Design review of the part built by this model. Coordinates are the model's own, in mm. A direction names the side the tool comes from. Coordinates: 2 decimals unless noted, no trailing zeros. Write each loop counter-clockwise with the first axis right and the second up, starting at its lowest first coordinate (ties: lowest second). Pieces come first, ordered by that corner, then holes.
Q1. Machinability: for faces 4 (the face through (-4, 1, 4)), 5 (the face through (2, 0, -2)), 6 (the face through (1.908, 12.601, -4.458)), 7 (the face through (2, 16, -2)), 8 (the face through (-5, 12, 2)), which of the approach directions +Z, -Z, +X, -X, +Y, -Y give a long, thin tool a straight path to every point of the face, cutting with its end or side? Answer none if there is none.
Q2. Add section B-B, the plane z = 0. Give the boundary of the cut face in (x, y), plus the area to 3 significant figures.
Q3. To check wall thickness, follow probe 1 along Y at (x, z) = (4.5, -5.5); probe 2 along X at (y, z) = (4.25, 0); probe 3 along X at (y, z) = (2.5, 0.5). State the ranges of each line that lie inside material, in increasing order.
Q4. Add section D-D, the plane y = 12. Give the boundary of the cut face in (x, z).
Q5. Add section C-C, the plane x = -5.75. Give the boundary of the cut face in (y, z).
Q6. Add section A-A, the plane x = 0. Give the boundary of the cut face in (y, z), plus the area to 3 significant figures.
Q7. Clearance check with flat-ended pins moving along their axes: pin 1 Ø3 at (x, z) = (0, 0) entering from +Y; pin 2 Ø4 at (y, z) = (7.5, 3) entering from -X; pin 3 Ø3 at (x, y) = (-3.5, 3.5) entering from -Z; pin 4 Ø1.5 at (x, y) = (1.5, 2) entering from -Z. State where each tip first meets the part, or that it passes through.
Q8. The part is to be moulded in two halves that separate along X. For faces 1 (the face through (-4, 8, 4)), 2 (the face through (0.33, 0.493, -7.493)), 3 (the face through (2.11, 8.11, 1.34)), say which applies: +X half, -X half, draft (parallel to the pull), parting line (faces both ways), or undercut.
from build123d import *

# Parameters (mm, degrees)
ESQUISSE1_R                  = 7.5
BOSS_EXTRU_1_DEPTH           = 16
ESQUISSE2_W                  = 2
ESQUISSE2_H                  = 7
ESQUISSE3_R                  = 2.5
ENL_V_MAT_EXTRU_1_DEPTH      = 16
ESQUISSE4_R                  = 2
ENL_V_MAT_EXTRU_2_DEPTH      = 20.19635382
R_P_TITION_CIRCULAIRE1_COUNT = 2
R_P_TITION_CIRCULAIRE1_ANGLE = 90


with BuildPart() as part:
    # Esquisse1 → Boss.-Extru.1 (new body)
    with BuildSketch(Plane(origin=(0, 0, 0), x_dir=(1, 0, 0), z_dir=(0, 1, 0))):
        with Locations(Location((0, 0, 0), (0, 0, 270))):
            Circle(ESQUISSE1_R)
    extrude(amount=BOSS_EXTRU_1_DEPTH)

    # Esquisse2 → Enlèvement de matière-Révolution1 (revolve, cut)
    with BuildSketch(Plane(origin=(0, 0, 0), x_dir=(0, 0, -1), z_dir=(1, 0, 0)), mode=Mode.PRIVATE) as enl_vement_de_mati_re_r_volution1_sk:
        with Locations((-6.5, 4.5)):
            Rectangle(ESQUISSE2_W, ESQUISSE2_H)
    revolve(enl_vement_de_mati_re_r_volution1_sk.sketch.rotate(Axis((0, 0, 0), (0, 1, 0)), 180), axis=Axis((0, 0, 0), (0, 1, 0)), mode=Mode.SUBTRACT)

    # Esquisse3 → Enlèv. mat.-Extru.1 (cut)
    with BuildSketch(Plane(origin=(0, 16, 0), x_dir=(1, 0, 0), z_dir=(0, 1, 0))):
        with Locations(Location((0, 0, 0), (0, 0, 270))):
            Circle(ESQUISSE3_R)
    extrude(amount=-ENL_V_MAT_EXTRU_1_DEPTH, mode=Mode.SUBTRACT)

    # Esquisse4 → Enlèv. mat.-Extru.2 (cut, through all)
    with BuildSketch(Plane.XY):
        with Locations((0, 12)):
            Circle(ESQUISSE4_R)
    enl_v_mat_extru_2 = extrude(amount=-ENL_V_MAT_EXTRU_2_DEPTH, mode=Mode.SUBTRACT)

    # Répétition circulaire1: Enlèv. mat.-Extru.2 ×2 about axis
    r_p_tition_circulaire1_axis = Axis((0, 16, 0), (0, 1, 0))
    for i in range(1, R_P_TITION_CIRCULAIRE1_COUNT):
        add(enl_v_mat_extru_2.rotate(r_p_tition_circulaire1_axis, i * R_P_TITION_CIRCULAIRE1_ANGLE / (R_P_TITION_CIRCULAIRE1_COUNT - 1)), mode=Mode.SUBTRACT)


solid = part.part
Here are the results:
1. face 4: none
1. face 5: +Z, -Z, +X, -X, -Y
1. face 6: -Z
1. face 7: +Z, -Z, +X, -X, +Y
1. face 8: -X
2. outline: (-7.5, 0) - (-2.5, 0) - (-2.5, 10) - (-7.5, 10) - (-7.5, 8) - (-5.5, 8) - (-5.5, 1) - (-7.5, 1) - close; (-7.5, 14) - (-2.5, 14) - (-2.5, 16) - (-7.5, 16) - close; (2.5, 0) - (7.5, 0) - (7.5, 1) - (5.5, 1) - (5.5, 8) - (7.5, 8) - (7.5, 16) - (2.5, 16) - close
2. area: 112 mm2
3. probe 1: y = 0 to 1, 8 to 16
3. probe 2: x = -5.5 to -2.5, 2.5 to 5.5
3. probe 3: x = -5.48 to -2.45, 2.45 to 5.48
4. outline: (-7.23, -2) arc R7.5 ccw to (-2, -7.23) - (-2, -2) - close; (-7.23, 2) - (-1.5, 2) arc R2.5 cw to (2, -1.5) - (2, -7.23) arc R7.5 ccw (long way) to start
5. outline: (0, -4.82) - (1, -4.82) - (1, 4.82) - (0, 4.82) - close; (8, -4.82) - (16, -4.82) - (16, 4.82) - (8, 4.82) - close; hole circle Ø4 at (12, 0)
6. outline: (0, -7.5) - (1, -7.5) - (1, -5.5) - (8, -5.5) - (8, -7.5) - (10, -7.5) - (10, -2.5) - (0, -2.5) - close; (0, 2.5) - (16, 2.5) - (16, 7.5) - (8, 7.5) - (8, 5.5) - (1, 5.5) - (1, 7.5) - (0, 7.5) - close; (14, -7.5) - (16, -7.5) - (16, -2.5) - (14, -2.5) - close
6. area: 112 mm2
7. pin 1: passes through
7. pin 2: stops at x = -7.42
7. pin 3: stops at z = -5.12
7. pin 4: stops at z = -5.45
8. face 1: draft
8. face 2: parting line
8. face 3: undercut
